Design review of the part built by this model. Coordinates are the model's own, in mm. A direction names the side the tool comes from. Coordinates: 2 decimals unless noted, no trailing zeros. Loops run counter-clockwise (first coordinate to the right, second up) from the corner with the lowest first, then second, coordinate; pieces in that order, holes last. Notation, with made-up numbers: (59.25, 0.25) -> (109.25, 0.25) arc R36 ccw to (109.25, 39.25) -> close; hole circle Ø11 at (3.5, 69). An arc over 180 degrees is marked (long way). Use CSV: the item, a comma, the result in double quotes.
Autodesk Inventor part; units mm, degrees
ref_plane "YZ Plane" through (0, 0, 0) normal (1, 0, 0) x (0, 1, 0)
ref_plane "XZ Plane" through (0, 0, 0) normal (0, 1, 0) x (-1, 0, 0)
ref_plane "XY Plane" through (0, 0, 0) normal (0, 0, 1) x (1, 0, 0)
sketch "Sketch1" plane through (0, 0, 0) normal (0, 0, 1) x (1, 0, 0)
  circle A0 centre (0, 0) radius 6.35
  dimension "d0" = 12.7
sketch "Sketch2" plane through (0, 0, 0) normal (0, 1, 0) x (-1, 0, 0)
  line L0 (0, 0) -> (0, -107.95)
  line L1 (12.7, -120.65) -> (228.6, -120.65)
  line L2 (241.3, -107.95) -> (241.3, 107.95)
  line L3 (228.6, 120.65) -> (12.7, 120.65)
  line L4 (0, 107.95) -> (0, 6.35)
  arc A0 (0, -107.95) -> (12.7, -120.65) centre (12.7, -107.95) ccw
  arc A1 (228.6, -120.65) -> (241.3, -107.95) centre (228.6, -107.95) ccw
  arc A2 (241.3, 107.95) -> (228.6, 120.65) centre (228.6, 107.95) ccw
  arc A3 (12.7, 120.65) -> (0, 107.95) centre (12.7, 107.95) ccw
  point P0 (0, -120.65)
  point P1 (241.3, -120.65)
  point P2 (241.3, 120.65)
  point P3 (0, 120.65)
  dimension "d1" = 6.35
  dimension "d2" = 120.65
  dimension "d3" = 241.3
  dimension "d4" = 241.3
  dimension "d8" = 12.7
sweep "Sweep1" add profiles "Sketch1" path "Sketch2"
properties part number "Ring_Of_Rebar" material "Steel"
Item 1: To check wall thickness, follow line 1 along X through (y, z) = (-0.75, -6.5); line 2 along Z through (x, y) = (-212, -4.75); line 3 along Z through (x, y) = (-98, 0). State the ranges of each line that lie inside material, in increasing order.
Checked values:
line 1,"-247.61 to -234.99, -6.31 to 6.31"
line 2,"-124.86 to -116.44, 116.44 to 124.86"
line 3,"-127 to -114.3, 114.3 to 127"
Item 2: Add section A-A (z = 22.5). Give the boundary of the cut face in (x, y).
Checked values:
outline,"circle Ø12.7 at (-241.3, 0); circle Ø12.7 at (0, 0)"
Item 3: Machinability: for faces 1 (the face through (0, 0, 0)), 2 (the face through (-122.161, -0.279, -114.306)), which of the approach directions +Z, -Z, +X, -X, +Y, -Y give a long, thin tool a straight path to every point of the face, cutting with its end or side? Answer none if there is none.
Checked values:
face 1,"+X, +Y, -Y"
face 2,"none"
Item 4: Draft analysis for pull direction X (two halves, no side actions). For faces 3 (the face through (-119.139, -0.279, 114.306)), 4 (the face through (0, 0, 6.35)), 5 (the face through (-1.38, 6.2, 56.44)), state which applies: pulls with the +X half, pulls with the -X half, needs draft (parallel to the pull), parting line crosses it, or undercut.
Checked values:
face 3,"undercut"
face 4,"needs draft"
face 5,"undercut"
Item 5: Clearance check with flat-ended pins moving along their axes: pin 1 (2 mm diameter, centred on y = 3, z = -26.5, fed in from +X); pin 2 (4 mm diameter, centred on x = 3, y = 1.5, fed in from -Z); pin 3 (4 mm diameter, centred on x = -2.5, y = -1, fed in from +Z). State where each tip first meets the part, or that it passes through.
Checked values:
pin 1,"x = 6.03"
pin 2,"z = -121.01"
pin 3,"z = 125.09"
Item 6: Add section C-C (x = -121.5). Give the boundary of the cut face in (y, z), then the cut area to 3 significant figures.
Checked values:
outline,"circle Ø12.7 at (0, -120.65); circle Ø12.7 at (0, 120.65)"
area,"253 mm^2"
Item 7: Add section B-B (y = 0). Give the boundary of the cut face in (x, z), then the cut area to 3 significant figures.
Checked values:
outline,"(-247.65, -107.95) arc R19.05 ccw to (-228.6, -127) -> (-12.7, -127) arc R19.05 ccw to (6.35, -107.95) -> (6.35, 0) -> (-6.35, 0) -> (-6.35, -107.95) arc R6.35 cw to (-12.7, -114.3) -> (-228.6, -114.3) arc R6.35 cw to (-234.95, -107.95) -> (-234.95, 107.95) arc R6.35 cw to (-228.6, 114.3) -> (-12.7, 114.3) arc R6.35 cw to (-6.35, 107.95) -> (-6.35, 6.35) -> (6.35, 6.35) -> (6.35, 107.95) arc R19.05 ccw to (-12.7, 127) -> (-228.6, 127) arc R19.05 ccw to (-247.65, 107.95) -> close"
area,"11,900 mm^2"
